```python
from build123d import *

# Parameters (mm, degrees)
SKETCH1_W           = 40
SKETCH1_H           = 40
BOSS_EXTRUDE1_DEPTH = 40
SKETCH2_W           = 10
SKETCH2_H           = 30
CUT_EXTRUDE1_DEPTH  = 40
SKETCH3_W           = 10
SKETCH3_H           = 10
CUT_EXTRUDE2_DEPTH  = 40
SKETCH4_W           = 30
SKETCH4_H           = 10
CUT_EXTRUDE3_DEPTH  = 30
SKETCH5_W           = 10
SKETCH5_H           = 10
CUT_EXTRUDE4_DEPTH  = 30
SKETCH6_W           = 20
SKETCH6_H           = 10
CUT_EXTRUDE6_DEPTH  = 10


with BuildPart() as part:
    # Sketch1 → Boss-Extrude1 (new body)
    with BuildSketch(Plane.XY):
        with Locations((20, 20)):
            Rectangle(SKETCH1_W, SKETCH1_H)
    extrude(amount=BOSS_EXTRUDE1_DEPTH)

    # Sketch2 → Cut-Extrude1 (cut)
    with BuildSketch(Plane.XY.offset(40)):
        with Locations((5, 25)):
            Rectangle(SKETCH2_W, SKETCH2_H)
        Polygon((0, 0), (10, 10), (0, 10), align=None)
    extrude(amount=-CUT_EXTRUDE1_DEPTH, mode=Mode.SUBTRACT)

    # Sketch3 → Cut-Extrude2 (cut)
    with BuildSketch(Plane.XZ):
        with Locations((5, 5)):
            Rectangle(SKETCH3_W, SKETCH3_H)
        with Locations((5, 35)):
            Rectangle(SKETCH3_W, SKETCH3_H)
    extrude(amount=-CUT_EXTRUDE2_DEPTH, mode=Mode.SUBTRACT)

    # Sketch4 → Cut-Extrude3 (cut)
    with BuildSketch(Plane(origin=(0, 40, 0), x_dir=(1, 0, 0), z_dir=(0, 1, 0))):
        with Locations((25, -35)):
            Rectangle(SKETCH4_W, SKETCH4_H)
    extrude(amount=-CUT_EXTRUDE3_DEPTH, mode=Mode.SUBTRACT)

    # Sketch5 → Cut-Extrude4 (cut)
    with BuildSketch(Plane(origin=(0, 40, 0), x_dir=(1, 0, 0), z_dir=(0, 1, 0))):
        with Locations((35, -25)):
            Rectangle(SKETCH5_W, SKETCH5_H)
    extrude(amount=-CUT_EXTRUDE4_DEPTH, mode=Mode.SUBTRACT)

    # Sketch6 → Cut-Extrude6 (cut)
    with BuildSketch(Plane.XY.offset(30)):
        with Locations((20, 35)):
            Rectangle(SKETCH6_W, SKETCH6_H)
    extrude(amount=-CUT_EXTRUDE6_DEPTH, mode=Mode.SUBTRACT)


solid = part.part
```
Verification items for the finished model (mm, model axes). A direction names the side the tool comes from. Coordinates: 2 decimals unless noted, no trailing zeros. Loops run counter-clockwise (first coordinate to the right, second up) from the corner with the lowest first, then second, coordinate; pieces in that order, holes last. Notation, with made-up numbers: (13.5, 27) - (45.5, 27) arc R26 ccw to (45.5, 49) - close; hole circle Ø7 at (48, 9). An arc over 180 degrees is marked (long way). Answer as a JSON object with one key per item and string values.
(1) Cross-section at C-C, the plane z = 21. Record the boundary of the cut face in (x, y).
Response:
{"outline": "(0, 0) - (40, 0) - (40, 10) - (30, 10) - (30, 30) - (10, 30) - (10, 10) - close"}
(2) Scan lines: line 1 along Y through (x, z) = (22.5, 38.5); line 2 along X through (y, z) = (7, 8); line 3 along X through (y, z) = (15, 21.5). Record each from-to range of solid material in increasing order.
Response:
{"line 1": "y = 0 to 10", "line 2": "x = 10 to 40", "line 3": "x = 10 to 30"}
(3) Cross-section at D-D, the plane y = 29. Record the boundary of the cut face in (x, z), then the cut area to 3 significant figures.
Response:
{"outline": "(10, 0) - (40, 0) - (40, 20) - (30, 20) - (30, 30) - (10, 30) - close", "area": "800 mm²"}
(4) Access from +Z, -Z, +X, -X, +Y, -Y to the whole of each face (thin tool, end or side, straight path). Record for faces 1 (the flat face through (20, 20, 30)), 2 (the flat face through (7, 3, 30)), 3 (the flat face through (25, 20, 0)), 4 (the flat face through (7, 3, 10)), 5 (the flat face through (30, 20, 25)).
Response:
{"face 1": "+Z, +X, -X, +Y", "face 2": "+Z, -X, +Y, -Y", "face 3": "-Z, +X, -X, +Y, -Y", "face 4": "-Z, -X, +Y, -Y", "face 5": "+Z, +X, +Y"}
(5) Mould release check, pull along X, two halves, no side actions. Record for faces 6 (the flat face through (40, 15, 15)), 7 (the flat face through (20, 30, 25)), 8 (the flat face through (10, 5, 35)): pulls with the +X half, pulls with the -X half, needs draft (parallel to the pull), parting line crosses it, or undercut.
Response:
{"face 6": "pulls with the +X half", "face 7": "needs draft", "face 8": "pulls with the -X half"}
(6) Cross-section at A-A, the plane x = 29. Record the boundary of the cut face in (y, z), then the cut area to 3 significant figures.
Response:
{"outline": "(0, 0) - (40, 0) - (40, 20) - (30, 20) - (30, 30) - (10, 30) - (10, 40) - (0, 40) - close", "area": "1,200 mm²"}
(7) Go/stop test with flat-tipped pins: pin 1 Ø12 at (y, z) = (20, 24) entering from -X; pin 2 Ø8 at (x, z) = (20, 23.5) entering from +Y; pin 3 Ø9 at (x, y) = (32, 27.5) entering from +Z; pin 4 Ø3 at (y, z) = (7.5, 28.5) entering from -X. Record where each tip stops, or that it passes through.
Response:
{"pin 1": "stops at x = 10", "pin 2": "stops at y = 40", "pin 3": "stops at z = 30", "pin 4": "stops at x = 6"}
(8) Cross-section at B-B, the plane y = 5.5. Record the boundary of the cut face in (x, z).
Response:
{"outline": "(5.5, 10) - (10, 10) - (10, 0) - (40, 0) - (40, 40) - (10, 40) - (10, 30) - (5.5, 30) - close"}
